```python
from build123d import *

# Parameters (mm, degrees)
BOSS_EXTRUDE1_DEPTH = 11.8
BOSS_EXTRUDE2_DEPTH = 4
CUT_EXTRUDE1_DEPTH  = 31.148507426
SKETCH4_R           = 2.3
BOSS_EXTRUDE4_DEPTH = 3.2


with BuildPart() as part:
    # Sketch1 → Boss-Extrude1 (new body)
    with BuildSketch(Plane.XY):
        Polygon((-11.25, 0), (11.25, 0), (11.25, 15.9), (15.95, 15.9), (15.95, 18.4), (11.25, 18.4), (11.25, 22.7), (-11.25, 22.7), (-11.25, 18.4), (-15.95, 18.4), (-15.95, 15.9), (-11.25, 15.9), align=None)
    extrude(amount=BOSS_EXTRUDE1_DEPTH)

    # Sketch2 → Boss-Extrude2 (add)
    with BuildSketch(Plane(origin=(0, 22.7, 0), x_dir=(1, 0, 0), z_dir=(0, 1, 0))):
        with BuildLine():
            Line((0.95, -8.4), (-0.005844314, -8.4))
            ThreePointArc((-0.005844314, -8.4), (-11.25, -5.9), (-0.005844314, -3.4))
            Line((-0.005844314, -3.4), (0.95, -3.4))
            ThreePointArc((0.95, -3.4), (3.45, -5.9), (0.95, -8.4))
        make_face()
    extrude(amount=BOSS_EXTRUDE2_DEPTH)

    # Sketch3 → Cut-Extrude1 (cut, through all)
    with BuildSketch(Plane(origin=(0, 22.7, 0), x_dir=(1, 0, 0), z_dir=(0, 1, 0))):
        with BuildLine():
            Line((-15.95, -5.25), (-14.409934208, -5.25))
            ThreePointArc((-14.409934208, -5.25), (-12.65, -5.9), (-14.409934208, -6.55))
            Line((-14.409934208, -6.55), (-15.95, -6.55))
            Line((-15.95, -6.55), (-15.95, -5.25))
        make_face()
        with BuildLine():
            Line((15.95, -6.55), (15.95, -5.25))
            Line((15.95, -5.25), (14.409934208, -5.25))
            ThreePointArc((14.409934208, -5.25), (12.65, -5.9), (14.409934208, -6.55))
            Line((14.409934208, -6.55), (15.95, -6.55))
        make_face()
    extrude(amount=-CUT_EXTRUDE1_DEPTH, mode=Mode.SUBTRACT)

    # Sketch4 → Boss-Extrude4 (add)
    with BuildSketch(Plane(origin=(0, 26.7, 0), x_dir=(1, 0, 0), z_dir=(0, 1, 0))):
        with Locations(Location((-5.35, -5.9, 0), (0, 0, 180))):
            Circle(SKETCH4_R)
    extrude(amount=BOSS_EXTRUDE4_DEPTH)


solid = part.part
```
For this review, take the finished solid that the model builds, in its own axes (mm). A direction names the side the tool comes from. Coordinates: 2 decimals unless noted, no trailing zeros. Loops run counter-clockwise (first coordinate to the right, second up) from the corner with the lowest first, then second, coordinate; pieces in that order, holes last.
1. Add section B-B, the plane z = 9. Give the boundary of the cut face in (x, y), then the cut area to 3 significant figures.
2. For faces 5 (the flat face through (-10, 22.7, 11)), 6 (the cylindrical face through (3.45, 24.67, 5.85)), 7 (the flat face through (-15, 17, 6.55)), 8 (the flat face through (-10, 22.7, 1)), 9 (the flat face through (15, 17, 5.25)), list the 3-axis set-ups (+Z, -Z, +X, -X, +Y, -Y) from which the entire face can be reached by the end or side of a thin tool; tool diameter is ignored.
3. Add section A-A, the plane x = -13.65. Give the boundary of the cut face in (y, z).
4. Add section D-D, the plane x = 6. Give the boundary of the cut face in (y, z).
5. Insertion check: P1, Ø4, axis at x = 14.5, z = 6, coming from the +Y side; P2, Ø6, axis at x = 1, z = 8, coming from the +Y side; P3, Ø1, axis at y = 15, z = 2.5, coming from the +X side. Each pin has a flat end and moves straight along its axis. Give the tip position at first contact, or say it passes through.
6. Add section C-C, the plane y = 16.5. Give the boundary of the cut face in (x, z), then the cut area to 3 significant figures.
7. Mouldability with a two-part tool opening along Z and no side actions: class faces 1 (the flat face through (15, 17, 6.55)), 2 (the flat face through (0.5, 24.7, 8.4)), 3 (the flat face through (-11.25, 8, 6)), 4 (the flat face through (0, 12, 0)) as +Z half, -Z half, draft (parallel to the pull), parting line (faces both ways), or undercut.
8. For line 1 (Z direction, x = -13.65, y = 17.3); line 2 (X direction, y = 17.35, z = 5.9); line 3 (Y direction, x = -12.5, z = 1), list the stretches that pass through material, from the lowest coordinate up.
Result:
1. outline: (-15.95, 15.9) - (-11.25, 15.9) - (-11.25, 0) - (11.25, 0) - (11.25, 15.9) - (15.95, 15.9) - (15.95, 18.4) - (11.25, 18.4) - (11.25, 22.7) - (-0.33, 22.7) - (-0.33, 26.7) - (-10.37, 26.7) - (-10.37, 22.7) - (-11.25, 22.7) - (-11.25, 18.4) - (-15.95, 18.4) - close
1. area: 574 mm2
2. face 5: +Z, -X, +Y
2. face 6: +X, +Y
2. face 7: -X, +Y, -Y
2. face 8: -Z, -X, +Y
2. face 9: +X, +Y, -Y
3. outline: (15.9, 0) - (18.4, 0) - (18.4, 4.9) - (15.9, 4.9) - close; (15.9, 6.9) - (18.4, 6.9) - (18.4, 11.8) - (15.9, 11.8) - close
4. outline: (0, 0) - (22.7, 0) - (22.7, 11.8) - (0, 11.8) - close
5. P1: stops at y = 18.4
5. P2: stops at y = 26.7
5. P3: stops at x = 11.25
6. outline: (-15.95, 0) - (15.95, 0) - (15.95, 5.25) - (14.41, 5.25) arc R1 cw (long way) to (14.41, 6.55) - (15.95, 6.55) - (15.95, 11.8) - (-15.95, 11.8) - (-15.95, 6.55) - (-14.41, 6.55) arc R1 cw (long way) to (-14.41, 5.25) - (-15.95, 5.25) - close
6. area: 367 mm2
7. face 1: undercut
7. face 2: +Z half
7. face 3: draft
7. face 4: -Z half
8. line 1: z = 0 to 4.9, 6.9 to 11.8
8. line 2: x = -12.65 to 12.65
8. line 3: y = 15.9 to 18.4
